```python
from build123d import *

# Parameters (mm, degrees)
BLOCK_SKETCH_W  = 15.9
BLOCK_SKETCH_H  = 15.9
BLOCK_DEPTH     = 7.95
ARM_SKETCH_W    = 8.586
ARM_SKETCH_H    = 24.05
SOCKET_SKETCH_W = 4.7625
SOCKET_SKETCH_H = 17.8


with BuildPart() as part:
    # Block Sketch → Block (new, symmetric)
    with BuildSketch(Plane.XY):
        with Locations((-18, 0)):
            Rectangle(BLOCK_SKETCH_W, BLOCK_SKETCH_H)
    extrude(amount=BLOCK_DEPTH, both=True)

    # Neck and Stud Sketch → Neck and Stud (revolve)
    with BuildSketch(Plane.XY, mode=Mode.PRIVATE) as neck_and_stud_sk:
        Polygon((9.5, 0), (9.5, 4.953), (0, 4.953), (0, 8.586), (-10.05, 8.586), (-10.05, 0), align=None)
    revolve(neck_and_stud_sk.sketch.rotate(Axis((-1000, 0, 0), (1, 0, 0)), 90), axis=Axis((-1000, 0, 0), (1, 0, 0)))

    # Arm Sketch → Arm (revolve)
    with BuildSketch(Plane.XY, mode=Mode.PRIVATE) as arm_sk:
        with Locations((-13.707, 19.975)):
            Rectangle(ARM_SKETCH_W, ARM_SKETCH_H)
    revolve(arm_sk.sketch.rotate(Axis((-18, 0, 0), (0, 1, 0)), 90), axis=Axis((-18, 0, 0), (0, 1, 0)))

    # Socket Sketch → Socket (revolve, cut)
    with BuildSketch(Plane.XY, mode=Mode.PRIVATE) as socket_sk:
        with Locations((-15.61875, 24.1)):
            Rectangle(SOCKET_SKETCH_W, SOCKET_SKETCH_H)
    revolve(socket_sk.sketch.rotate(Axis((-18, 0, 0), (0, 1, 0)), 90), axis=Axis((-18, 0, 0), (0, 1, 0)), mode=Mode.SUBTRACT)


solid = part.part
```
Input: part model. Units: mm. Frame: model coordinates. A direction names the side the tool comes from. Give positions to 0.01 mm unless a question says otherwise; leave off trailing zeros. Order: outer loops, then holes, each group sorted by start corner. A loop starts at its lowest first (then second) coordinate and runs counter-clockwise, first axis right, second up.
1. Cut plane D-D (y = 25.5). Return loops of the section in (x, z) (1 decimal).
Computed:
outline: circle Ø17.2 at (-18, 0); hole circle Ø9.5 at (-18, 0)
2. Pin query (flat end, axial travel): pin 1 Ø1.5 at (x, z) = (-23, -6.5) entering from -Y; pin 2 Ø8 at (y, z) = (3, -1.5) entering from -X; pin 3 Ø8 at (x, y) = (-18, 3) entering from -Z; pin 4 Ø3 at (x, y) = (-16.5, 14) entering from +Z. Return the tip coordinate at first contact, or that it passes through.
Computed:
pin 1: stops at y = -7.95
pin 2: stops at x = -25.95
pin 3: stops at z = -7.95
pin 4: stops at z = 8.59
3. Cut plane B-B (z = 0). Return loops of the section in (x, y).
Computed:
outline: (-26.59, 7.95) - (-25.95, 7.95) - (-25.95, -7.95) - (-10.05, -7.95) - (-10.05, -8.59) - (0, -8.59) - (0, -4.95) - (9.5, -4.95) - (9.5, 4.95) - (0, 4.95) - (0, 8.59) - (-9.41, 8.59) - (-9.41, 32) - (-13.24, 32) - (-13.24, 15.2) - (-22.76, 15.2) - (-22.76, 32) - (-26.59, 32) - close
4. Cut plane C-C (y = 0). Return loops of the section in (x, z).
Computed:
outline: (-25.95, -7.95) - (-10.05, -7.95) - (-10.05, -8.59) - (0, -8.59) - (0, -4.95) - (9.5, -4.95) - (9.5, 4.95) - (0, 4.95) - (0, 8.59) - (-10.05, 8.59) - (-10.05, 7.95) - (-25.95, 7.95) - close
5. Set-up query: faces 4 (the face through (-25.95, 0, 0)), 5 (the face through (-18, 15.2, 0)), 6 (the face through (-25, 7.95, -7)), 7 (the face through (-18, 0, -7.95)), 8 (the face through (-5.095, 8.382, -1.861)). Return all of +Z, -Z, +X, -X, +Y, -Y with unobstructed straight access to the full face (end or side cutting, diameter ignored); none if empty.
Computed:
face 4: +Z, -Z, -X, -Y
face 5: +Y
face 6: -Z, -X, +Y
face 7: -Z, -X, -Y
face 8: +X
6. Cut plane A-A (x = -18). Return loops of the section in (y, z), and give its area (3 significant figures).
Computed:
outline: (-7.95, -7.95) - (7.95, -7.95) - (7.95, -8.59) - (32, -8.59) - (32, -4.76) - (15.2, -4.76) - (15.2, 4.76) - (32, 4.76) - (32, 8.59) - (7.95, 8.59) - (7.95, 7.95) - (-7.95, 7.95) - close
area: 506 mm2
7. Draft query along Z for faces 1 (the face through (-18, 0, 7.95)), 2 (the face through (-10.05, 7, 7)), 3 (the face through (-13.35, 23.72, 1.03)). Return one class per face: released by +Z, released by -Z, zero draft, split by the parting line, or undercut.
Computed:
face 1: released by +Z
face 2: zero draft
face 3: undercut
8. Line query: probe 1 along X at (y, z) = (21, 0); probe 2 along X at (y, z) = (-3.5, 5.25); probe 3 along X at (y, z) = (24, -2.5). Output: solid intervals per line, ascending.
Computed:
probe 1: x = -26.59 to -22.76, -13.24 to -9.41
probe 2: x = -25.95 to 0
probe 3: x = -26.21 to -22.05, -13.95 to -9.79
